Autodesk Inventor part; units mm, degrees
ref_plane "YZ Plane" through (0, 0, 0) normal (1, 0, 0) x (0, 1, 0)
ref_plane "XZ Plane" through (0, 0, 0) normal (0, 1, 0) x (-1, 0, 0)
ref_plane "XY Plane" through (0, 0, 0) normal (0, 0, 1) x (1, 0, 0)
sketch "Sketch1" plane through (0, 0, 0) normal (0, 0, 1) x (1, 0, 0)
  line L0 (0, 0) -> (25.4, 0)
  line L1 (25.4, 0) -> (25.4, 50.8)
  line L2 (25.4, 50.8) -> (0, 50.8)
  line L3 (0, 50.8) -> (0, 0)
  line L4 (1.5875, 49.2125) -> (23.8125, 49.2125)
  line L5 (23.8125, 49.2125) -> (23.8125, 1.5875)
  line L6 (23.8125, 1.5875) -> (1.5875, 1.5875)
  line L7 (1.5875, 1.5875) -> (1.5875, 49.2125)
  dimension "d0" = 25.4
  dimension "d1" = 50.8
  dimension "d2" = 1.5875
extrude "Extrusion1" add sketch "Sketch1" along normal blind 76.2
sketch "Sketch3" plane through (25.4, 0, 0) normal (1, 0, 0) x (0, 0, -1)
  line L0 (0, 50.8) -> (-76.2, 50.8) construction
  line L1 (-38.1, 50.8) -> (-38.1, 25.4) construction
  circle A0 centre (-38.1, 25.4) radius 7.493
  point P0 (0, 0)
  dimension "d10" = 25.4
  dimension "d15" = 14.986
extrude "Extrusion3" cut sketch "Sketch3" against normal blind 82.55
sketch "Sketch4" plane through (0, 50.8, 0) normal (0, 1, 0) x (1, 0, 0)
  line L0 (1.5875, 0) -> (23.8125, 0) construction
  line L1 (12.7, 0) -> (12.7, -12.7) construction
  line L2 (23.8125, -76.2) -> (1.5875, -76.2) construction
  line L3 (12.7, -76.2) -> (12.7, -63.5) construction
  circle A0 centre (12.7, -63.5) radius 2.5797
  circle A1 centre (12.7, -12.7) radius 2.5797
  point P0 (0, 0)
  dimension "d16" = 12.7
  dimension "d17" = 12.7
  dimension "d18" = 5.1594
extrude "Extrusion4" cut sketch "Sketch4" against normal blind 82.55
sketch "Sketch5" plane through (25.4, 0, 0) normal (1, 0, 0) x (0, 0, -1)
  line L0 (0, 0) -> (0, 50.8)
  line L1 (0, 25.4) -> (-12.7, 25.4) construction
  line L2 (-76.2, 49.2125) -> (-76.2, 1.5875)
  line L3 (-76.2, 25.4) -> (-63.5, 25.4) construction
  circle A0 centre (-63.5, 25.4) radius 2.5797
  circle A1 centre (-12.7, 25.4) radius 2.5797
  dimension "d21" = 12.7
  dimension "d22" = 12.7
  dimension "d23" = 5.1594
extrude "Extrusion5" cut sketch "Sketch5" against normal blind 25.4
properties part number "1x1 Bumper Attachment"
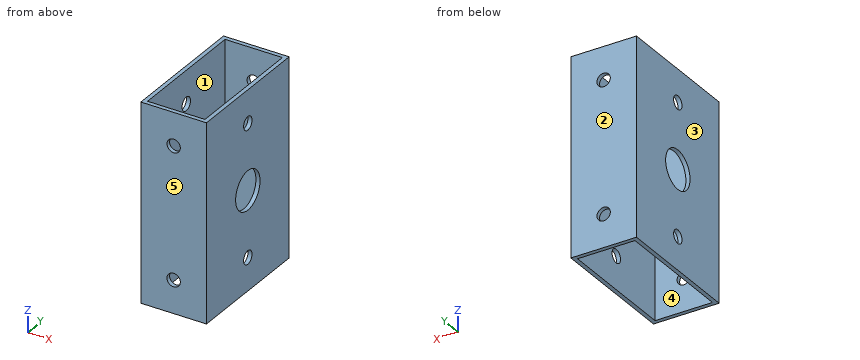
Design review of the part built by this model. Coordinates are the model's own, in mm. Face numbers are marked on the shaded views. A direction names the side the tool comes from. Give positions to 0.01 mm unless a question says otherwise; leave off trailing zeros. Loops run counter-clockwise (first coordinate to the right, second up) from the corner with the lowest first, then second, coordinate; pieces in that order, holes last. Notation, with made-up numbers: M -2,8 L 20,8 A24 cw 20,24 Z; hole C 27.25,-28 d10. An arc over 180 degrees is marked long. Return JSON: item names as keys, results as strings. Group by question number.
Item 1: We need section D-D (x = 12.7). Give the boundary of the cut face in (y, z), and give its area (3 significant figures).
Item 2: We need section B-B (y = 39). Give the boundary of the cut face in (x, z).
Item 3: Tool access review of the marked faces 1 and 2: name each direction out of +Z, -Z, +X, -X, +Y, -Y from which nothing blocks a thin tool from reaching the whole face with its end or side.
Item 4: Mouldability with a two-part tool opening along X and no side actions: class the marked faces 3, 4 and 5 as released by +X, released by -X, zero draft, split by the parting line, or undercut.
Item 5: For probe 1 along Z at (x, y) = (12.7, 50.3); probe 2 along Y at (x, z) = (24.45, 12.7); probe 3 along Y at (x, z) = (17.75, 24), list the stretches that pass through material, from the lowest coordinate up.
Item 6: We need section A-A (z = 12.7). Give the boundary of the cut face in (x, y).
Item 7: Insertion check: pin 1 Ø4.5 at (y, z) = (25.4, 12.7) entering from +X. The pin has a flat end and moves straight along its axis. Give the tip position at first contact, or say it passes through.
Item 8: We need section C-C (z = 38.1). Give the boundary of the cut face in (x, y).
Output:
{
 "1": {"outline": "M 0,0 L 1.59,0 L 1.59,10.12 L 0,10.12 Z; M 0,15.28 L 1.59,15.28 L 1.59,60.92 L 0,60.92 Z; M 0,66.08 L 1.59,66.08 L 1.59,76.2 L 0,76.2 Z; M 49.21,0 L 50.8,0 L 50.8,10.12 L 49.21,10.12 Z; M 49.21,15.28 L 50.8,15.28 L 50.8,60.92 L 49.21,60.92 Z; M 49.21,66.08 L 50.8,66.08 L 50.8,76.2 L 49.21,76.2 Z", "area": "209 mm^2"},
 "2": {"outline": "M 0,0 L 1.59,0 L 1.59,76.2 L 0,76.2 Z; M 23.81,0 L 25.4,0 L 25.4,76.2 L 23.81,76.2 Z"},
 "3": {"face 1": "+Z, -Z", "face 2": "+Z, -Z, +X, -X, +Y"},
 "4": {"face 3": "released by -X", "face 4": "undercut", "face 5": "zero draft"},
 "5": {"probe 1": "z = 0 to 10.12, 15.28 to 60.92, 66.08 to 76.2", "probe 2": "y = 0 to 22.82, 27.98 to 50.8", "probe 3": "y = 0 to 1.59, 49.21 to 50.8"},
 "6": {"outline": "M 0,0 L 10.12,0 L 10.12,1.59 L 1.59,1.59 L 1.59,22.82 L 0,22.82 Z; M 0,27.98 L 1.59,27.98 L 1.59,49.21 L 10.12,49.21 L 10.12,50.8 L 0,50.8 Z; M 15.28,0 L 25.4,0 L 25.4,22.82 L 23.81,22.82 L 23.81,1.59 L 15.28,1.59 Z; M 15.28,49.21 L 23.81,49.21 L 23.81,27.98 L 25.4,27.98 L 25.4,50.8 L 15.28,50.8 Z"},
 "7": {"pin 1": "passes through"},
 "8": {"outline": "M 0,0 L 25.4,0 L 25.4,17.91 L 23.81,17.91 L 23.81,1.59 L 1.59,1.59 L 1.59,17.91 L 0,17.91 Z; M 0,32.89 L 1.59,32.89 L 1.59,49.21 L 23.81,49.21 L 23.81,32.89 L 25.4,32.89 L 25.4,50.8 L 0,50.8 Z"}
}
